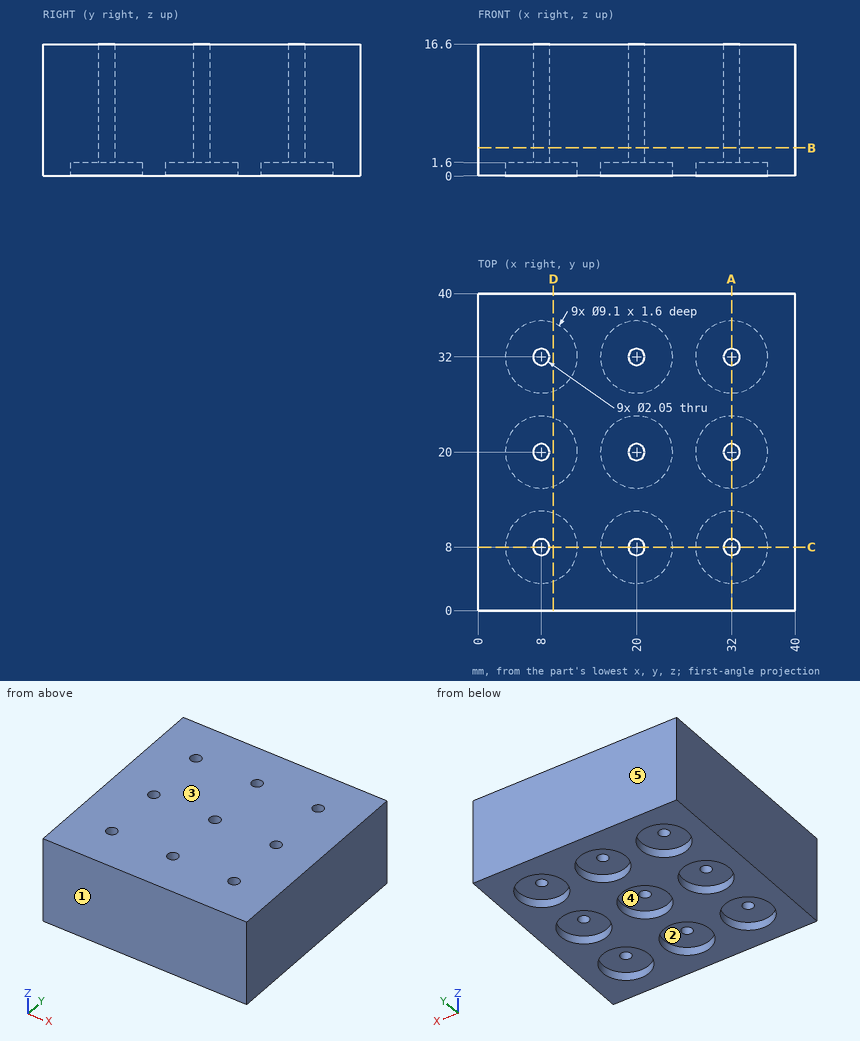
The drawing under review shows one solid part. Ordinate dimensions are in mm from its lowest x, y, z. A direction names the side the tool comes from. Coordinates: 2 decimals unless noted, no trailing zeros. Loops run counter-clockwise (first coordinate to the right, second up) from the corner with the lowest first, then second, coordinate; pieces in that order, holes last. Notation, with made-up numbers: (12.25, -1.5) - (65.25, -1.5) arc R15 cw to (65.25, 20.5) - close; hole circle Ø9 at (85, 43). An arc over 180 degrees is marked (long way). Return JSON: item names as keys, results as strings.
Item 1: For line 1 (Y direction, x = 32, z = 12) (3 decimals); line 2 (X direction, y = 19.5, z = 9), list the stretches that pass through material, from the lowest coordinate up.
Determined:
{"line 1": "y = 0 to 6.975, 9.025 to 18.975, 21.025 to 30.975, 33.025 to 40", "line 2": "x = 0 to 7.11, 8.89 to 19.11, 20.89 to 31.11, 32.89 to 40"}
Item 2: Insertion check: pin 1 (4.5 mm diameter, centred on x = 21.5, y = 31.5, fed in from -Z). The pin has a flat end and moves straight along its axis. Give the tip position at first contact, or say it passes through.
Determined:
{"pin 1": "stops at z = 1.6"}
Item 3: Mouldability with a two-part tool opening along Y and no side actions: class the marked faces 3, 4 and 5 as pulls with the +Y half, pulls with the -Y half, needs draft (parallel to the pull), parting line crosses it, or undercut.
Determined:
{"face 3": "needs draft", "face 4": "undercut", "face 5": "pulls with the +Y half"}
Item 4: Take a section at B-B (z = 3.5). State how many separate pieces and enclosed holes the cut face has, then the cut area to 3 significant figures.
Determined:
{"separate pieces": "1", "enclosed holes": "9", "area": "1,570 mm2"}
Item 5: For the marked faces 1 and 2, list the 3-axis set-ups (+Z, -Z, +X, -X, +Y, -Y) from which the entire face can be reached by the end or side of a thin tool; tool diameter is ignored.
Determined:
{"face 1": "+Z, -Z, +X, -X, -Y", "face 2": "-Z"}
Item 6: Take a section at D-D (x = 9.5). Give the boundary of the cut face in (y, z).
Determined:
{"outline": "(0, 0) - (3.7, 0) - (3.7, 1.6) - (12.3, 1.6) - (12.3, 0) - (15.7, 0) - (15.7, 1.6) - (24.3, 1.6) - (24.3, 0) - (27.7, 0) - (27.7, 1.6) - (36.3, 1.6) - (36.3, 0) - (40, 0) - (40, 16.6) - (0, 16.6) - close"}
Item 7: Take a section at A-A (x = 32). Give the boundary of the cut face in (y, z) (3 decimals).
Determined:
{"outline": "(0, 0) - (3.45, 0) - (3.45, 1.6) - (6.975, 1.6) - (6.975, 16.6) - (0, 16.6) - close; (9.025, 1.6) - (12.55, 1.6) - (12.55, 0) - (15.45, 0) - (15.45, 1.6) - (18.975, 1.6) - (18.975, 16.6) - (9.025, 16.6) - close; (21.025, 1.6) - (24.55, 1.6) - (24.55, 0) - (27.45, 0) - (27.45, 1.6) - (30.975, 1.6) - (30.975, 16.6) - (21.025, 16.6) - close; (33.025, 1.6) - (36.55, 1.6) - (36.55, 0) - (40, 0) - (40, 16.6) - (33.025, 16.6) - close"}
